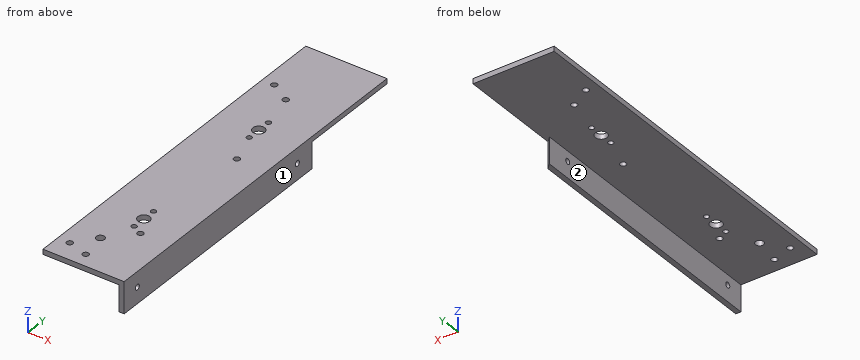
```python
from build123d import *

# Parameters (mm, degrees)
BOSS_EXTRUDE1_DEPTH     = 203.2
CUT_EXTRUDE2_DEPTH      = 20.685
SKETCH5_R               = 3.683
SKETCH5_R_2             = 1.63195
CUT_EXTRUDE3_DEPTH      = 20.685
SKETCH6_R               = 1.7526
CUT_EXTRUDE4_DEPTH      = 51.8
SKETCH8_R               = 1.89865
CUT_EXTRUDE5_DEPTH      = 4.175
SKETCH9_R               = 1.89865
CUT_EXTRUDE6_DEPTH      = 4.175
BOSS_EXTRUDE2_DEPTH     = 3.175
SKETCH11_R              = 2.54
CUT_EXTRUDE7_DEPTH      = 20.685
SKETCH12_R              = 1.89865
CUT_EXTRUDE8_DEPTH      = 4.175
SKETCH13_R              = 3.683
SKETCH13_R_2            = 1.63195
CUT_EXTRUDE9_DEPTH      = 1
CUT_EXTRUDE9_DEPTH_BACK = 20.685


with BuildPart() as part:
    # Sketch1 → Boss-Extrude1 (new body)
    with BuildSketch(Plane(origin=(0, 0, 0), x_dir=(1, 0, 0), z_dir=(0, 1, 0))):
        Polygon((0, 0), (-50.8, 0), (-50.8, 3.175), (-3.175, 3.175), (-3.175, 19.685), (0, 19.685), align=None)
    extrude(amount=BOSS_EXTRUDE1_DEPTH)

    # Sketch4 → Cut-Extrude2 (cut, through all)
    with BuildSketch(Plane.XY):
        Polygon((-50.8, 214.122), (-57.250524058, 214.122), (-57.250524058, 247.071987418), (14.491605927, 247.071987418), (14.491605927, 163.322), (0, 163.322), align=None)
    extrude(amount=-CUT_EXTRUDE2_DEPTH, mode=Mode.SUBTRACT)

    # Sketch5 → Cut-Extrude3 (cut, through all)
    with BuildSketch(Plane.XY):
        with Locations((-25.4, 152.4)):
            Circle(SKETCH5_R)
        with Locations((-25.4, 160.782)):
            Circle(SKETCH5_R_2)
        with Locations((-25.4, 144.018)):
            Circle(SKETCH5_R_2)
    extrude(amount=-CUT_EXTRUDE3_DEPTH, mode=Mode.SUBTRACT)

    # Sketch6 → Cut-Extrude4 (cut, through all)
    with BuildSketch(Plane(origin=(0, 0, 0), x_dir=(0, 0, -1), z_dir=(1, 0, 0))):
        with Locations((9.530474513, 11.43)):
            Circle(SKETCH6_R)
        with Locations((9.530474513, 150.622)):
            Circle(SKETCH6_R)
    extrude(amount=-CUT_EXTRUDE4_DEPTH, mode=Mode.SUBTRACT)

    # Sketch8 → Cut-Extrude5 (cut, through all)
    with BuildSketch(Plane(origin=(0, 0, -3.175), x_dir=(-1, 0, 0), z_dir=(0, 0, -1))):
        with Locations((30.48, 8.89)):
            Circle(SKETCH8_R)
        with Locations((30.48, 182.88)):
            Circle(SKETCH8_R)
    extrude(amount=-CUT_EXTRUDE5_DEPTH, mode=Mode.SUBTRACT)

    # Sketch9 → Cut-Extrude6 (cut, through all)
    with BuildSketch(Plane(origin=(0, 0, -3.175), x_dir=(-1, 0, 0), z_dir=(0, 0, -1))):
        with Locations((19.05, 40.64)):
            Circle(SKETCH9_R)
        with Locations((19.05, 124.46)):
            Circle(SKETCH9_R)
    extrude(amount=-CUT_EXTRUDE6_DEPTH, mode=Mode.SUBTRACT)

    # Sketch10 → Boss-Extrude2 (add)
    with BuildSketch(Plane.XY):
        Polygon((0, 228.6), (0, 163.322), (-39.878, 203.2), (-50.8, 203.2), (-50.8, 228.6), align=None)
    extrude(amount=-BOSS_EXTRUDE2_DEPTH)

    # Sketch11 → Cut-Extrude7 (cut, through all)
    with BuildSketch(Plane.XY):
        with Locations((-33.136196499, 25.4)):
            Circle(SKETCH11_R)
    extrude(amount=-CUT_EXTRUDE7_DEPTH, mode=Mode.SUBTRACT)

    # Sketch12 → Cut-Extrude8 (cut, through all)
    with BuildSketch(Plane(origin=(0, 0, -3.175), x_dir=(-1, 0, 0), z_dir=(0, 0, -1))):
        with Locations((43.18, 12.7)):
            Circle(SKETCH12_R)
        with Locations((43.18, 190.498941664)):
            Circle(SKETCH12_R)
    extrude(amount=-CUT_EXTRUDE8_DEPTH, mode=Mode.SUBTRACT)

    # Sketch13 → Cut-Extrude9 (cut, two sides)
    with BuildSketch(Plane.XY) as cut_extrude9_sk:
        with Locations((-25.4, 52.4)):
            Circle(SKETCH13_R)
        with Locations((-25.4, 60.782)):
            Circle(SKETCH13_R_2)
        with Locations((-25.4, 44.018)):
            Circle(SKETCH13_R_2)
    extrude(amount=CUT_EXTRUDE9_DEPTH, mode=Mode.SUBTRACT)
    extrude(cut_extrude9_sk.sketch, amount=-CUT_EXTRUDE9_DEPTH_BACK, mode=Mode.SUBTRACT)


solid = part.part
```
For this review, take the finished solid that the model builds, in its own axes (mm). Face numbers are marked on the shaded views. A direction names the side the tool comes from. Round coordinates to 2 decimals unless told otherwise and drop trailing zeros. Write each loop counter-clockwise with the first axis right and the second up, starting at its lowest first coordinate (ties: lowest second). Pieces come first, ordered by that corner, then holes. Notation, with made-up numbers: M 77,-37 L 98,-37 A24 cw 98,-18 Z; hole C -5.75,-13.75 d11. An arc over 180 degrees is marked long. One line per item, written item: value. Start each with the question number.
(1) We need section C-C (y = 25.4). Give the boundary of the cut face in (x, z) (3 decimals).
(2) We need section B-B (y = 52.4). Give the boundary of the cut face in (x, z) (3 decimals), and give its area (3 significant figures).
(3) We need section D-D (z = -13.5). Give the boundary of the cut face in (x, y) (3 decimals).
(4) Wall thickness on line 1 (Y direction, x = -43, z = -1.25); line 2 (Y direction, x = -30.48, z = -0.85); line 3 (X direction, y = 16, z = -18.5) (3 decimals): over which ranges is each line inside the solid? List them lowest first.
(5) Machinability: for the marked faces 1 and 2, which of the approach directions +Z, -Z, +X, -X, +Y, -Y give a long, thin tool a straight path to every point of the face, cutting with its end or side? Answer none if there is none.
(6) Insertion check: pin 1 (6 mm diameter, centred on x = -30.48, y = 8.89, fed in from +Z); pin 2 (5 mm diameter, centred on x = -25.4, y = 44.018, fed in from -Z) (3 decimals); pin 3 (1 mm diameter, centred on y = 155.5, z = -10, fed in from -X) (3 decimals); pin 4 (3 mm diameter, centred on x = -33.14, y = 25.4, fed in from +Z). Each pin has a flat end and moves straight along its axis. Give the tip position at first contact, or say it passes through.
(7) We need section A-A (x = -43.18). Give the boundary of the cut face in (y, z) (3 decimals), and give its area (3 significant figures).
Result:
1. outline: M -50.8,-3.175 L -35.676,-3.175 L -35.676,0 L -50.8,0 Z; M -30.596,-3.175 L -3.175,-3.175 L -3.175,-19.685 L 0,-19.685 L 0,0 L -30.596,0 Z
2. outline: M -50.8,-3.175 L -29.083,-3.175 L -29.083,0 L -50.8,0 Z; M -21.717,-3.175 L -3.175,-3.175 L -3.175,-19.685 L 0,-19.685 L 0,0 L -21.717,0 Z
2. area: 190 mm²
3. outline: M -3.175,0 L 0,0 L 0,163.322 L -3.175,166.497 Z
4. line 1: 0 to 10.81, 14.59 to 188.61, 192.39 to 228.6
4. line 2: 0 to 6.99, 10.79 to 180.98, 184.78 to 228.6
4. line 3: -3.175 to 0
5. face 1: +Z, -Z, +X, +Y, -Y
5. face 2: -Z, -X, +Y, -Y
6. pin 1: z = 0
6. pin 2: z = -3.175
6. pin 3: x = -3.175
6. pin 4: through
7. outline: M 0,-3.175 L 10.801,-3.175 L 10.801,0 L 0,0 Z; M 14.599,-3.175 L 188.6,-3.175 L 188.6,0 L 14.599,0 Z; M 192.398,-3.175 L 228.6,-3.175 L 228.6,0 L 192.398,0 Z
7. area: 702 mm²
